Drawing for the job (mm, zero at the part's lowest x, y, z). A direction names the side the tool comes from. Coordinates: 2 decimals unless noted, no trailing zeros. Write each loop counter-clockwise with the first axis right and the second up, starting at its lowest first coordinate (ties: lowest second). Pieces come first, ordered by that corner, then holes. Notation, with made-up numbers: (41.5, -7.75) -> (71.5, -7.75) arc R24 ccw to (71.5, 5.25) -> close; hole circle Ø4 at (72, 27). An arc over 180 degrees is marked (long way). Write item = value, one per line. Start each with the question number.
Q1. Band-saw the part on B-B, the plane y = 72.5. List the corners of the cut face in (x, z), plus the area to 3 significant figures.
Q2. Probe line 1 (Y direction, x = 83, z = 37) (1 decimal); line 2 (Y direction, x = 13.5, z = 50.5) (1 decimal); line 3 (Z direction, x = 36.5, y = 49). List the from-to ranges inside material, lowest first.
Q3. Tool access for the marked faces 1, 2 and 3: list every direction of +Z, -Z, +X, -X, +Y, -Y with a clear straight run to the whole face (end or side of a thin tool).
Q4. Pull direction Y, two halves, no side cores. Call the marked faces 4, 5 and 6: released by +Y, released by -Y, zero draft, split by the parting line, or undercut.
Q5. Band-saw the part on D-D, the plane z = 47.5. List the corners of the cut face in (x, y), plus the area to 3 significant figures.
Q6. Band-saw the part on C-C, the plane x = 66.5. List the corners of the cut face in (y, z) (1 decimal), plus the area to 3 significant figures.
Q7. Band-saw the part on A-A, the plane z = 37.5. List the corners of the cut face in (x, y).
Q8. Pin check, flat tips, straight feed: P1, Ø8, axis at x = 119.5, y = 127.5, coming from the +Z side (1 decimal); P2, Ø8, axis at y = 31.5, z = 37.5, coming from the +X side (1 decimal); P3, Ø6, axis at x = 105.5, y = 116.5, coming from the +Z side (1 decimal). Stop position of each tip, or through.
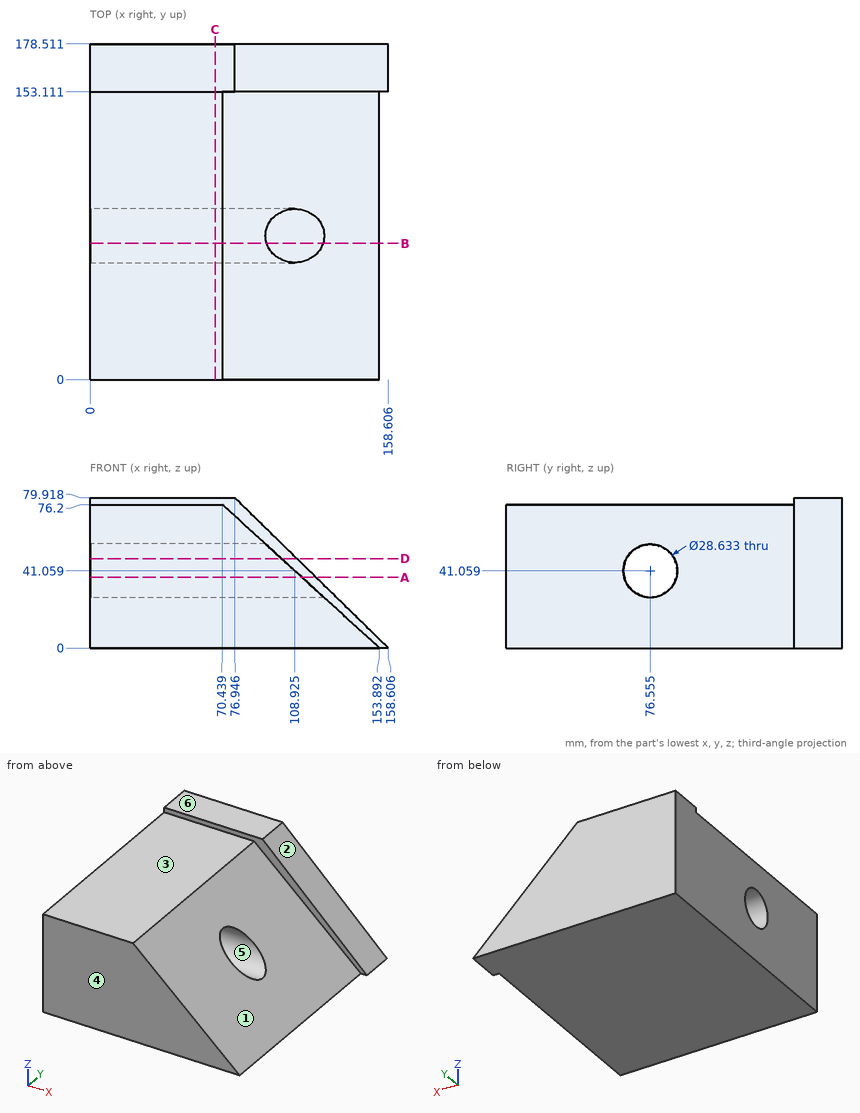
Ans:
q1.outline = (0, 0) -> (153.89, 0) -> (123.96, 27.33) -> (0, 27.33) -> close; (0, 54.79) -> (93.89, 54.79) -> (70.44, 76.2) -> (0, 76.2) -> close
q1.area = 5,560 mm2
q2.line_1 = 0 to 62.8, 90.3 to 178.5
q2.line_2 = 0 to 65.8, 87.3 to 178.5
q2.line_3 = 0 to 76.2
q3.face_1 = +Z, +X, -Y
q3.face_2 = +Z, +X, +Y, -Y
q3.face_3 = +Z, +X, -X, -Y
q4.face_4 = released by -Y
q4.face_5 = undercut
q4.face_6 = zero draft
q5.outline = (0, 0) -> (101.87, 0) -> (101.87, 63.77) -> (0, 63.77) -> close; (0, 89.34) -> (101.87, 89.34) -> (101.87, 153.11) -> (110.07, 153.11) -> (110.07, 178.51) -> (0, 178.51) -> close
q5.area = 15,800 mm2
q6.outline = (0, 0) -> (178.5, 0) -> (178.5, 79.9) -> (153.1, 79.9) -> (153.1, 76.2) -> (0, 76.2) -> close; hole circle Ø28.6 at (76.6, 41.1)
q6.area = 13,100 mm2
q7.outline = (0, 0) -> (112.82, 0) -> (112.82, 62.69) -> (0, 62.69) -> close; (0, 90.42) -> (112.82, 90.42) -> (112.82, 153.11) -> (120.29, 153.11) -> (120.29, 178.51) -> (0, 178.51) -> close
q8.P1 = 35.1
q8.P2 = 117.2
q8.P3 = 46.9
